Here's how the part is built. I have some questions about the finished solid (model axes, mm). A direction names the side the tool comes from. Give positions to 0.01 mm unless a question says otherwise; leave off trailing zeros. Order: outer loops, then holes, each group sorted by start corner. A loop starts at its lowest first (then second) coordinate and runs counter-clockwise, first axis right, second up. Notation, with made-up numbers: M 57,53 L 66,53 A27 ccw 66,89 Z; hole C 5.25,33.5 d4. An arc over 180 degrees is marked long. Use one line per item in the form item = value.
Autodesk Inventor part; units mm, degrees
ref_plane "YZ Plane" through (0, 0, 0) normal (1, 0, 0) x (0, 1, 0)
ref_plane "XY Plane" through (0, 0, 0) normal (0, 0, 1) x (1, 0, 0)
sketch "Sketch1" plane through (0, 0, 0) normal (0, 0, 1) x (1, 0, 0)
  arc A0 (3.8578, 24.2337) -> (23.4537, 24.2337) centre (13.6558, 26.2337) ccw
  arc A1 (28.3527, 48.2337) -> (-1.0412, 48.2337) centre (13.6558, 51.2337) ccw
  line L0 (-1.0412, 48.2337) -> (3.8578, 24.2337)
  line L1 (28.3527, 48.2337) -> (23.4537, 24.2337)
  dimension "d32" = 20
  dimension "d33" = 30
extrude "Extrusion8" add sketch "Sketch1" along normal blind 7
sketch "Sketch8" plane through (0, 0, 7) normal (0, 0, 1) x (1, 0, 0)
  arc A0 (28.3527, 48.2337) -> (-1.0412, 48.2337) centre (13.6558, 51.2337) ccw
  circle A1 centre (13.6558, 51.2337) radius 5
  point P0 (0, 0)
  dimension "d36" = 10
extrude "Extrusion9" add sketch "Sketch8" along normal blind 40
ref_plane "Work Plane8" through (13.6558, 56.2337, 7) normal (0, 1, 0) x (-1, 0, 0)
sketch "Sketch13" plane through (0, 0, 0) normal (0, 0, -1) x (-1, 0, 0)
  circle A0 centre (-13.6558, 51.2337) radius 5
  circle A1 centre (-13.6558, 51.2337) radius 5
  point P0 (0, 0)
hole "Hole1" at (13.6558, 51.2337, 0) direction (0, 0, 1) diameter 6 end through all counterbore diameter 8 counterbore depth 7
sketch "Sketch14" plane through (13.6558, 51.2337, 47) normal (0, 0, 1) x (1, 0, 0)
  circle A0 centre (0, 0) radius 4
  arc A1 (14.6969, -3) -> (-14.6969, -3) centre (0, 0) ccw
  circle A2 centre (0, 0) radius 5
  point P0 (-13.6558, -51.2337)
  dimension "d52" = 8
extrude "Extrusion11" cut sketch "Sketch14" against normal blind 13
sketch "Sketch15" plane through (13.6558, 56.2337, 7) normal (0, 1, 0) x (-1, 0, 0)
  line L0 (5, 10) -> (-5.1311, 10)
  line L1 (4, 40) -> (-4, 40)
  point P0 (13.6558, -7)
  dimension "d55" = 30
bend part "Bend Part3" radius 10 angle 90 line through (8.6558, 56.2337, 17) along (1, 0, 0) centre toward (0, 1, 0) moving side (0, 0, 1) both sides no
properties part number "Vòi"
Q1. I need wall thicknesses on L1, parallel to X at y = 69.5, z = 32; L2, parallel to Z at x = 15.5, y = 62.5; L3, parallel to Z at x = 8.5, y = 19.5. Which ranges of each line are inside material? Lowest first, please.
Found:
L1 = 9.66 to 10.66, 16.66 to 17.66
L2 = 0 to 7, 26.66 to 29.07, 33.96 to 36.29
L3 = 0 to 7
Q2. I want a section at D-D on y = 25.5. Write out the boundary of the cut face in (x, z).
Found:
outline = M 3.6,0 L 23.71,0 L 23.71,7 L 3.6,7 Z
Q3. Thinking about a two-plate mould opening in X: for faces 1 (the face through (1.374, 36.402, 3.451)), 2 (the face through (11, 53, 7)), 3 (the face through (25.937, 36.402, 3.451)), 4 (the face through (14.805, 54.005, 12.07)), which applies, +X half, -X half, draft (parallel to the pull), parting line (faces both ways), or undercut?
Found:
face_1 = -X half
face_2 = undercut
face_3 = +X half
face_4 = undercut
Q4. On a 3-axis mill with a long thin cutter (end or side, diameter ignored), from which of +Z, -Z, +X, -X, +Y, -Y can I reach the whole of each face in a straight line? I mean faces 5 (the face through (16.344, 47.018, 11.93)), 6 (the face through (12.454, 55.049, 3.549)), 7 (the face through (15, 67.526, 28)), 8 (the face through (15, 80.526, 29)), 9 (the face through (13, 42, 0)). Say none if no direction works.
Found:
face_5 = none
face_6 = -Z
face_7 = +Y
face_8 = +Z, -Z, +X, -X, +Y
face_9 = -Z, +X, -X, +Y, -Y
Q5. I want a section at C-C on x = 2. Write out the boundary of the cut face in (y, z), then the cut area to 3 significant figures.
Found:
outline = M 33.33,0 L 60.68,0 L 60.68,7 L 33.33,7 Z
area = 191 mm²
Q6. I'm going to push flat-ended pins straight in: pin 1 Ø1.5 at (x, y) = (7, 41.5) entering from +Z; pin 2 Ø1.5 at (y, z) = (54, 10) entering from -X; pin 3 Ø6.5 at (x, y) = (13.66, 51.23) entering from -Z. Where does each tip first touch, or does it pass through?
Found:
pin_1 = 7
pin_2 = 9.08
pin_3 = 7
Q7. I want a section at A-A on x = 14.5. Write out the boundary of the cut face in (y, z), then the cut area to 3 significant figures.
Found:
outline = M 16.27,0 L 47.32,0 L 47.32,7 L 48.35,7 L 48.35,17 A17.88 cw 66.23,34.88 L 80.53,34.88 L 80.53,35.91 L 67.53,35.91 L 67.53,36.93 L 66.23,36.93 A19.93 ccw 46.31,17 L 46.31,7 L 16.27,7 Z; M 54.11,7 L 55.14,7 L 55.14,0 L 66.21,0 L 66.21,7 L 56.16,7 L 56.16,17 A10.07 cw 66.23,27.07 L 67.53,27.07 L 67.53,28.09 L 80.53,28.09 L 80.53,29.12 L 66.23,29.12 A12.12 ccw 54.11,17 Z
area = 465 mm²
Q8. I want a section at B-B on z = 5.5. Write out the boundary of the cut face in (x, y), then the cut area to 3 significant figures.
Found:
outline = M -1.04,48.23 L 3.86,24.23 A10 ccw 23.45,24.23 L 28.35,48.23 A15 ccw long Z; hole C 13.66,51.23 d8
area = 1,100 mm²
